```python
from build123d import *

# Parameters (mm, degrees)
SKETCH1_R               = 25.4
SKETCH1_R_2             = 23.8125
BOSS_EXTRUDE1_DEPTH     = 158.75
CUT_EXTRUDE1_DEPTH      = 163.763271348
CUT_EXTRUDE1_DEPTH_BACK = 163.763271348
CUT_EXTRUDE2_DEPTH      = 163.763271348
CUT_EXTRUDE2_DEPTH_BACK = 163.763271348


with BuildPart() as part:
    # Sketch1 → Boss-Extrude1 (new body)
    with BuildSketch(Plane(origin=(0, 0, 0), x_dir=(1, 0, 0), z_dir=(0, 1, 0))):
        with Locations(Location((0, 0, 0), (0, 0, 90))):
            Circle(SKETCH1_R)
        with Locations(Location((0, 0, 0), (0, 0, 90))):
            Circle(SKETCH1_R_2, mode=Mode.SUBTRACT)
    extrude(amount=BOSS_EXTRUDE1_DEPTH)

    # Sketch2 → Cut-Extrude1 (cut, two sides: drawn at the far end of the back side and taken through both)
    with BuildSketch(Plane.XY.offset(-CUT_EXTRUDE1_DEPTH_BACK)):
        Polygon((25.4, 133.35), (25.4, 158.75), (-0.960093291, 166.540490079), (-25.4, 158.75), (-25.4, 133.35), (0, 158.75), align=None)
    extrude(amount=CUT_EXTRUDE1_DEPTH + CUT_EXTRUDE1_DEPTH_BACK, mode=Mode.SUBTRACT)

    # Sketch3 → Cut-Extrude2 (cut, two sides: drawn at the far end of the back side and taken through both)
    with BuildSketch(Plane(origin=(0, 0, 0), x_dir=(0, 0, -1), z_dir=(1, 0, 0)).offset(-CUT_EXTRUDE2_DEPTH_BACK)):
        Polygon((-25.4, 25.4), (-25.4, 0), (0.032632353, -12.112837501), (25.4, 0), (25.4, 25.4), (0, 0), align=None)
    extrude(amount=CUT_EXTRUDE2_DEPTH + CUT_EXTRUDE2_DEPTH_BACK, mode=Mode.SUBTRACT)


solid = part.part
```
The model under review builds one solid part; all positions refer to its coordinate system, in mm. Round coordinates to 2 decimals unless told otherwise and drop trailing zeros. Loops run counter-clockwise (first coordinate to the right, second up) from the corner with the lowest first, then second, coordinate; pieces in that order, holes last. Notation, with made-up numbers: M 77,88.5 L 101,88.5 A21 cw 101,99.5 Z; hole C 1,43 d7. An arc over 180 degrees is marked long. Write item = value, one per line.
Item 1: Insertion check: P1, Ø2, axis at x = 13.5, y = 136, coming from the -Z side; P2, Ø2, axis at y = 105, z = 14.5, coming from the +X side; P3, Ø2, axis at y = 99, z = 11.5, coming from the +X side. Each pin has a flat end and moves straight along its axis. Give the tip position at first contact, or say it passes through.
Return value:
P1 = -22.11
P2 = 21.52
P3 = 23.13
Item 2: For line 1 (X direction, y = 67.5, z = 0); line 2 (Z direction, x = -1, y = 105.5); line 3 (Z direction, x = -5, y = 60.5), list the stretches that pass through material, from the lowest coordinate up. Write a range as [from, to].
Return value:
line_1 = [-25.4, -23.81], [23.81, 25.4]
line_2 = [-25.38, -23.79], [23.79, 25.38]
line_3 = [-24.9, -23.28], [23.28, 24.9]
Item 3: Take a section at A-A on z = -6.5. Write out the cut boundary in (x, y).
Return value:
outline = M -24.55,6.5 L -22.91,6.5 L -22.91,135.84 L -24.55,134.2 Z; M 22.91,6.5 L 24.55,6.5 L 24.55,134.2 L 22.91,135.84 Z
Item 4: Take a section at C-C on y = 61. Write out the cut boundary in (x, z) (1 decimal), then the cut area to 3 significant figures.
Return value:
outline = C 0,0 d50.8; hole C 0,0 d47.6
area = 245 mm2
Item 5: The part is to be moulded in two halves that separate along X. For faces 1 (the flat face through (0, 24, 24)), 2 (the cylindrical face through (-7.629, 78.264, -24.227)), 3 (the flat face through (23.93, 134.82, 1.76)), 4 (the cylindrical face through (-7.2, 78.3, -22.7)), say which applies: released by +X, released by -X, zero draft, split by the parting line, or undercut.
Return value:
face_1 = zero draft
face_2 = split by the parting line
face_3 = released by +X
face_4 = undercut
Item 6: Take a section at B-B on x = -22. Write out the cut boundary in (y, z).
Return value:
outline = M 9.11,-9.11 L 12.69,-12.69 L 136.75,-12.69 L 136.75,-9.11 Z; M 9.11,9.11 L 136.75,9.11 L 136.75,12.69 L 12.69,12.69 Z
